Geometry: final body of the model. Coordinates: model frame, mm. Face numbers are marked on the shaded views. A direction names the side the tool comes from. Give positions to 0.01 mm unless a question says otherwise; leave off trailing zeros. Loops run counter-clockwise (first coordinate to the right, second up) from the corner with the lowest first, then second, coordinate; pieces in that order, holes last. Notation, with made-up numbers: (42.5, 87.5) - (99.5, 87.5) arc R24 cw to (99.5, 119.5) - close; hole circle Ø2 at (70.25, -20). An arc over 180 degrees is marked (long way). Use CSV: the item, a comma, the result in double quotes. Start each with the question number.
```python
from build123d import *

# Parameters (mm, degrees)
SKETCH_1_W          = 35
SKETCH_1_H          = 40
EXTRUDE_1_DEPTH     = 4
SKETCH_2_R          = 1.6
CUT_EXTRUDE_1_DEPTH = 6
SKETCH_3_W          = 35
SKETCH_3_H          = 5
EXTRUDE_2_DEPTH     = 21
SKETCH_4_R          = 1.6
CUT_EXTRUDE_2_DEPTH = 15
SKETCH_5_R          = 2.8
CUT_EXTRUDE_3_DEPTH = 2
SKETCH_6_W          = 40
SKETCH_6_H          = 10
EXTRUDE_3_DEPTH     = 5
SKETCH_7_W          = 35
SKETCH_7_H          = 5
EXTRUDE_4_DEPTH     = 10


with BuildPart() as part:
    # 草图1 → 凸台-拉伸1 (new body)
    with BuildSketch(Plane(origin=(0, 0, 0), x_dir=(1, 0, 0), z_dir=(0, 1, 0))):
        with Locations((17.5, 20)):
            Rectangle(SKETCH_1_W, SKETCH_1_H)
    extrude(amount=EXTRUDE_1_DEPTH)

    # 草图2 → 切除-拉伸1 (cut)
    with BuildSketch(Plane(origin=(0, 4, 0), x_dir=(1, 0, 0), z_dir=(0, 1, 0))):
        with Locations((10.6, 29.5)):
            Circle(SKETCH_2_R)
        with Locations((20.6, 29.5)):
            Circle(SKETCH_2_R)
        with Locations((20.6, 10.5)):
            Circle(SKETCH_2_R)
        with Locations((10.6, 10.5)):
            Circle(SKETCH_2_R)
    extrude(amount=-CUT_EXTRUDE_1_DEPTH, mode=Mode.SUBTRACT)

    # 草图3 → 凸台-拉伸2 (add)
    with BuildSketch(Plane.XZ):
        with Locations((17.5, -37.5)):
            Rectangle(SKETCH_3_W, SKETCH_3_H)
    extrude(amount=EXTRUDE_2_DEPTH)

    # 草图4 → 切除-拉伸2 (cut)
    with BuildSketch(Plane(origin=(0, 0, -40), x_dir=(-1, 0, 0), z_dir=(0, 0, -1))):
        with Locations((-10, -16)):
            Circle(SKETCH_4_R)
        with Locations((-20, -16)):
            Circle(SKETCH_4_R)
    extrude(amount=-CUT_EXTRUDE_2_DEPTH, mode=Mode.SUBTRACT)

    # 草图5 → 切除-拉伸3 (cut)
    with BuildSketch(Plane(origin=(0, 0, -40), x_dir=(-1, 0, 0), z_dir=(0, 0, -1))):
        with Locations((-20, -16)):
            Circle(SKETCH_5_R)
        with Locations((-10, -16)):
            Circle(SKETCH_5_R)
    extrude(amount=-CUT_EXTRUDE_3_DEPTH, mode=Mode.SUBTRACT)

    # 草图6 → 凸台-拉伸3 (add)
    with BuildSketch(Plane(origin=(0, 0, -40), x_dir=(-1, 0, 0), z_dir=(0, 0, -1))):
        with Locations((-55, -16)):
            Rectangle(SKETCH_6_W, SKETCH_6_H)
    extrude(amount=-EXTRUDE_3_DEPTH)

    # 草图7 → 凸台-拉伸4 (add)
    with BuildSketch(Plane.XZ):
        with Locations((17.5, -2.5)):
            Rectangle(SKETCH_7_W, SKETCH_7_H)
    extrude(amount=EXTRUDE_4_DEPTH)


solid = part.part
```
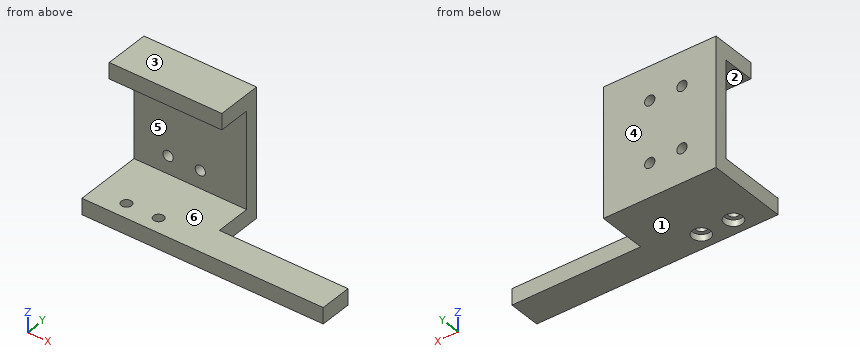
Item 1: Mould query, pull axis Z, two halves, no side actions, for the marked faces 3, 4, 5 and 6. Classes: pulls with the +Z half, pulls with the -Z half, needs draft (parallel to the pull), parting line crosses it, or undercut.
Item 2: Section D-D (x = 20). Output: boundary loops of the cut face in (y, z), plus the area to 3 significant figures.
Item 3: Pin query (flat end, axial travel): pin 1 Ø4 at (x, z) = (15.5, -2.5) entering from -Y; pin 2 Ø4 at (x, y) = (20, -16) entering from -Z; pin 3 Ø5 at (x, y) = (60.5, -11.5) entering from +Z. Return the tip coordinate at first contact, or that it passes through.
Item 4: Section B-B (z = -10.5). Output: boundary loops of the cut face in (x, y), plus the area to 3 significant figures.
Item 5: Section C-C (y = -7.25). Output: boundary loops of the cut face in (x, z), plus the area to 3 significant figures.
Item 6: Ray query, probe 1 along X at (y, z) = (2, -10.5); probe 2 along Z at (x, y) = (10.6, 2.4); probe 3 along Z at (x, y) = (9, -2.25). Return the intervals inside material, ascending.
Item 7: Section A-A (y = -16). Output: boundary loops of the cut face in (x, z).
Item 8: Reachability of the marked faces 1 and 2 from +Z, -Z, +X, -X, +Y, -Y: full face, straight path, thin tool, end or side. Return the list, or none.
Outcome:
1,face 3,"pulls with the +Z half"
1,face 4,"needs draft"
1,face 5,"undercut"
1,face 6,"undercut"
2,outline,"(-21, -40) - (-18.8, -40) - (-18.8, -38) - (-17.6, -38) - (-17.6, -35) - (-21, -35) - close; (-14.4, -38) - (-13.2, -38) - (-13.2, -40) - (4, -40) - (4, -30.98) - (0, -30.98) - (0, -35) - (-14.4, -35) - close; (-10, -5) - (0, -5) - (0, -9.02) - (4, -9.02) - (4, 0) - (-10, 0) - close; (0, -28.02) - (4, -28.02) - (4, -11.98) - (0, -11.98) - close"
2,area,"270 mm2"
3,pin 1,"stops at y = -10"
3,pin 2,"stops at z = -38"
3,pin 3,"stops at z = -35"
4,outline,"(0, 0) - (9, 0) - (9, 4) - (0, 4) - close; (12.2, 0) - (19, 0) - (19, 4) - (12.2, 4) - close; (22.2, 0) - (35, 0) - (35, 4) - (22.2, 4) - close"
4,area,"114 mm2"
5,outline,"(0, -40) - (35, -40) - (35, -35) - (0, -35) - close; (0, -5) - (35, -5) - (35, 0) - (0, 0) - close"
5,area,"350 mm2"
6,probe 1,"x = 0 to 9, 12.2 to 19, 22.2 to 35"
6,probe 2,"z = -40 to -31.1, -27.9 to -12.1, -8.9 to 0"
6,probe 3,"z = -40 to -35, -5 to 0"
7,outline,"(0, -40) - (7.2, -40) - (7.2, -38) - (8.4, -38) - (8.4, -35) - (0, -35) - close; (11.6, -38) - (12.8, -38) - (12.8, -40) - (17.2, -40) - (17.2, -38) - (18.4, -38) - (18.4, -35) - (11.6, -35) - close; (21.6, -38) - (22.8, -38) - (22.8, -40) - (75, -40) - (75, -35) - (21.6, -35) - close"
8,face 1,"-Z, +X, -X, +Y, -Y"
8,face 2,"+X, -X, -Y"
